```python
from build123d import *

# Parameters (mm, degrees)
SKETCH1_R                = 3.175
BOSS_EXTRUDE1_DEPTH      = 950
M5_CLEARANCE_HOLE1_D     = 5.3
M5_CLEARANCE_HOLE1_DEPTH = 5
M5_CLEARANCE_HOLE1_TIP   = 1.59228064
M5X0_8_TAPPED_HOLE1_D    = 4.2


with BuildPart() as part:
    # Sketch1 → Boss-Extrude1 (new body)
    with BuildSketch(Plane.XZ):
        with BuildLine():
            Line((77, 0), (3, 0))
            ThreePointArc((3, 0), (0.878679656, -0.878679656), (0, -3))
            Line((0, -3), (0, -17))
            ThreePointArc((0, -17), (0.878679656, -19.121320344), (3, -20))
            Line((3, -20), (14.5, -20))
            ThreePointArc((14.5, -20), (15.560660172, -19.560660172), (16, -18.5))
            Line((16, -18.5), (16, -17.5))
            ThreePointArc((16, -17.5), (15.560660172, -16.439339828), (14.5, -16))
            Line((14.5, -16), (13.2, -16))
            Line((13.2, -16), (13.2, -16.5))
            Line((13.2, -16.5), (10.75, -16.5))
            ThreePointArc((10.75, -16.5), (10.219669914, -16.280330086), (10, -15.75))
            Line((10, -15.75), (10, -12.810660172))
            ThreePointArc((10, -12.810660172), (10.057090351, -12.523647598), (10.219669914, -12.280330086))
            Line((10.219669914, -12.280330086), (13.108757211, -9.391242789))
            ThreePointArc((13.108757211, -9.391242789), (14.649768118, -8.361572221), (16.467514421, -8))
            Line((16.467514421, -8), (23.532485579, -8))
            ThreePointArc((23.532485579, -8), (25.350231882, -8.361572221), (26.891242789, -9.391242789))
            Line((26.891242789, -9.391242789), (29.780330086, -12.280330086))
            ThreePointArc((29.780330086, -12.280330086), (29.942909649, -12.523647598), (30, -12.810660172))
            Line((30, -12.810660172), (30, -15.75))
            ThreePointArc((30, -15.75), (29.780330086, -16.280330086), (29.25, -16.5))
            Line((29.25, -16.5), (26.8, -16.5))
            Line((26.8, -16.5), (26.8, -16))
            Line((26.8, -16), (25.5, -16))
            ThreePointArc((25.5, -16), (24.439339828, -16.439339828), (24, -17.5))
            Line((24, -17.5), (24, -18.5))
            ThreePointArc((24, -18.5), (24.439339828, -19.560660172), (25.5, -20))
            Line((25.5, -20), (54.5, -20))
            ThreePointArc((54.5, -20), (55.560660172, -19.560660172), (56, -18.5))
            Line((56, -18.5), (56, -17.5))
            ThreePointArc((56, -17.5), (55.560660172, -16.439339828), (54.5, -16))
            Line((54.5, -16), (53.2, -16))
            Line((53.2, -16), (53.2, -16.5))
            Line((53.2, -16.5), (50.75, -16.5))
            ThreePointArc((50.75, -16.5), (50.219669914, -16.280330086), (50, -15.75))
            Line((50, -15.75), (50, -12.810660172))
            ThreePointArc((50, -12.810660172), (50.057090351, -12.523647598), (50.219669914, -12.280330086))
            Line((50.219669914, -12.280330086), (53.108757211, -9.391242789))
            ThreePointArc((53.108757211, -9.391242789), (54.649768118, -8.361572221), (56.467514421, -8))
            Line((56.467514421, -8), (63.532485579, -8))
            ThreePointArc((63.532485579, -8), (65.350231882, -8.361572221), (66.891242789, -9.391242789))
            Line((66.891242789, -9.391242789), (69.780330086, -12.280330086))
            ThreePointArc((69.780330086, -12.280330086), (69.942909649, -12.523647598), (70, -12.810660172))
            Line((70, -12.810660172), (70, -15.75))
            ThreePointArc((70, -15.75), (69.780330086, -16.280330086), (69.25, -16.5))
            Line((69.25, -16.5), (66.8, -16.5))
            Line((66.8, -16.5), (66.8, -16))
            Line((66.8, -16), (65.5, -16))
            ThreePointArc((65.5, -16), (64.439339828, -16.439339828), (64, -17.5))
            Line((64, -17.5), (64, -18.5))
            ThreePointArc((64, -18.5), (64.439339828, -19.560660172), (65.5, -20))
            Line((65.5, -20), (77, -20))
            ThreePointArc((77, -20), (79.121320344, -19.121320344), (80, -17))
            Line((80, -17), (80, -3))
            ThreePointArc((80, -3), (79.121320344, -0.878679656), (77, 0))
        make_face()
        with Locations(Location((6, -6, 0), (0, 0, 270))):
            Circle(SKETCH1_R, mode=Mode.SUBTRACT)
        with Locations(Location((74, -6, 0), (0, 0, 270))):
            Circle(SKETCH1_R, mode=Mode.SUBTRACT)
        with BuildLine():
            Line((7.45, -18.5), (4.3, -18.5))
            ThreePointArc((4.3, -18.5), (2.320101013, -17.679898987), (1.5, -15.7))
            Line((1.5, -15.7), (1.5, -12.75))
            ThreePointArc((1.5, -12.75), (1.719669914, -12.219669914), (2.25, -12))
            Line((2.25, -12), (7.45, -12))
            ThreePointArc((7.45, -12), (7.980330086, -12.219669914), (8.2, -12.75))
            Line((8.2, -12.75), (8.2, -17.75))
            ThreePointArc((8.2, -17.75), (7.980330086, -18.280330086), (7.45, -18.5))
        make_face(mode=Mode.SUBTRACT)
        with BuildLine():
            Line((54.546446609, -3.853553391), (41.9, -16.5))
            Line((41.9, -16.5), (38.1, -16.5))
            Line((38.1, -16.5), (25.453553391, -3.853553391))
            ThreePointArc((25.453553391, -3.853553391), (25.345167015, -3.308658284), (25.807106781, -3))
            Line((25.807106781, -3), (54.192893219, -3))
            ThreePointArc((54.192893219, -3), (54.654832985, -3.308658284), (54.546446609, -3.853553391))
        make_face(mode=Mode.SUBTRACT)
        with BuildLine():
            Line((71.8, -17.75), (71.8, -12.75))
            ThreePointArc((71.8, -12.75), (72.019669914, -12.219669914), (72.55, -12))
            Line((72.55, -12), (77.75, -12))
            ThreePointArc((77.75, -12), (78.280330086, -12.219669914), (78.5, -12.75))
            Line((78.5, -12.75), (78.5, -15.7))
            ThreePointArc((78.5, -15.7), (77.679898987, -17.679898987), (75.7, -18.5))
            Line((75.7, -18.5), (72.55, -18.5))
            ThreePointArc((72.55, -18.5), (72.019669914, -18.280330086), (71.8, -17.75))
        make_face(mode=Mode.SUBTRACT)
    extrude(amount=-BOSS_EXTRUDE1_DEPTH)

    # M5 Clearance Hole1
    with Locations(Plane.XY):
        with Locations((48, 15), (48, 35), (48, 65), (32, 65), (32, 35), (32, 15)):
            Hole(M5_CLEARANCE_HOLE1_D / 2, depth=M5_CLEARANCE_HOLE1_DEPTH)
            with Locations((0, 0, -(M5_CLEARANCE_HOLE1_DEPTH + M5_CLEARANCE_HOLE1_TIP / 2))):  # 118° drill point
                Cone(0, M5_CLEARANCE_HOLE1_D / 2, M5_CLEARANCE_HOLE1_TIP, mode=Mode.SUBTRACT)

    # M5x0.8 Tapped Hole1 (through all)
    with Locations(Plane(origin=(0, 0, -20), x_dir=(-1, 0, 0), z_dir=(0, 0, -1))):
        with Locations((-40, 64.001015899)):
            Hole(M5X0_8_TAPPED_HOLE1_D / 2)


solid = part.part
```
Geometry check sheet. Reference: the model listing, model coordinates, mm. Coordinates: 2 decimals unless noted, no trailing zeros.
Q1. Depth check by flat-ended pin: pin 1 Ø10 at (x, z) = (54.5, -12) entering from +Y; pin 2 Ø5.5 at (x, y) = (61, 247.5) entering from -Z (3 decimals); pin 3 Ø5 at (x, y) = (32, 35) entering from +Z; pin 4 Ø3 at (x, y) = (32, 65) entering from +Z. Enter the tip coordinate at first touch or a pass-through.
Reply:
pin 1: stops at y = 950
pin 2: stops at z = -8.005
pin 3: stops at z = -7.9
pin 4: stops at z = -8.9
Q2. Sectioned sample at A-A on y = 423. Give the number of separate pieces and of enclosed holes in the cut face, and give its area (3 significant figures).
Reply:
separate pieces: 1
enclosed holes: 5
area: 862 mm2
Q3. Thickness scan on probe 1 along Y at (x, z) = (48, -2.2); probe 2 along Z at (x, y) = (73, 657); probe 3 along Z at (x, y) = (74.5, 450). Record the ranges inside material, lowest first.
Reply:
probe 1: y = 0 to 12.35, 17.65 to 32.35, 37.65 to 62.35, 67.65 to 950
probe 2: z = -20 to -18.5, -12 to -9.01, -2.99 to 0
probe 3: z = -20 to -18.5, -12 to -9.14, -2.86 to 0
Q4. Draft check along X on faces 1 (the face through (41, 468, 0)), 2 (the face through (40, 468, -3)). Enter one of: released by +X, released by -X, zero draft, split by the parting line, or undercut.
Reply:
face 1: zero draft
face 2: undercut
